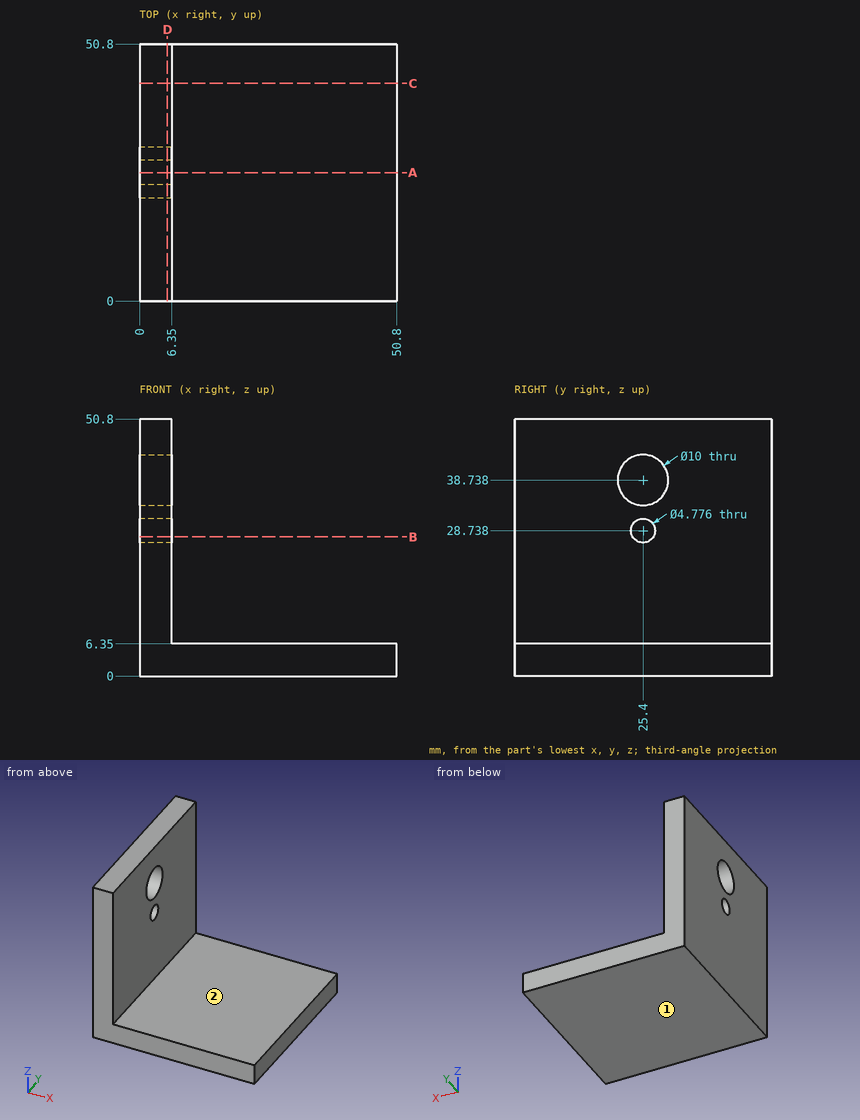
Design review of the part shown in the three views and the two pictorial views. Dimensions are in mm from the part's minimum x, y and z. A direction names the side the tool comes from. Give positions to 0.01 mm unless a question says otherwise; leave off trailing zeros. Loops run counter-clockwise (first coordinate to the right, second up) from the corner with the lowest first, then second, coordinate; pieces in that order, holes last. Notation, with made-up numbers: M -12,9.25 L 28,9.25 A12 cw 28,28.25 Z; hole C -5,79.25 d1. An arc over 180 degrees is marked long. Answer as a JSON object with one key per item and string values.
Item 1: Wall thickness on line 1 along Z through (x, y) = (4.5, 25.4); line 2 along Z through (x, y) = (43, 43): over which ranges is each line inside the solid? List them lowest first.
Output values:
{"line 1": "z = 0 to 26.35, 31.13 to 33.74, 43.74 to 50.8", "line 2": "z = 0 to 6.35"}
Item 2: We need section A-A (y = 25.4). State the section outline as (x, z) points.
Output values:
{"outline": "M 0,0 L 50.8,0 L 50.8,6.35 L 6.35,6.35 L 6.35,26.35 L 0,26.35 Z; M 0,31.13 L 6.35,31.13 L 6.35,33.74 L 0,33.74 Z; M 0,43.74 L 6.35,43.74 L 6.35,50.8 L 0,50.8 Z"}
Item 3: We need section B-B (z = 27.5). State the section outline as (x, y) points.
Output values:
{"outline": "M 0,0 L 6.35,0 L 6.35,23.36 L 0,23.36 Z; M 0,27.44 L 6.35,27.44 L 6.35,50.8 L 0,50.8 Z"}
Item 4: We need section C-C (y = 43). State the section outline as (x, z) points.
Output values:
{"outline": "M 0,0 L 50.8,0 L 50.8,6.35 L 6.35,6.35 L 6.35,50.8 L 0,50.8 Z"}
Item 5: We need section D-D (x = 5.5). State the section outline as (y, z) points, and give its area (3 significant figures).
Output values:
{"outline": "M 0,0 L 50.8,0 L 50.8,50.8 L 0,50.8 Z; hole C 25.4,38.74 d10; hole C 25.4,28.74 d4.78", "area": "2,480 mm2"}
Item 6: For P1, Ø22, axis at x = 23, y = 27.5, coming from the +Z side; P2, Ø12, axis at y = 32, z = 31.5, coming from the +X side; P3, Ø4.5, axis at y = 25.4, z = 28.74, coming from the +X side, all flat-tipped, find the tip position at first contact; note any pin that passes through.
Output values:
{"P1": "stops at z = 6.35", "P2": "stops at x = 6.35", "P3": "passes through"}
Item 7: Machinability: for the marked faces 1 and 2, which of the approach directions +Z, -Z, +X, -X, +Y, -Y give a long, thin tool a straight path to every point of the face, cutting with its end or side? Answer none if there is none.
Output values:
{"face 1": "-Z, +X, -X, +Y, -Y", "face 2": "+Z, +X, +Y, -Y"}
